Source: CAD feature listing. Evaluate the final solid. Frame: model axes, mm. A direction names the side the tool comes from. Give positions to 0.01 mm unless a question says otherwise; leave off trailing zeros. Order: outer loops, then holes, each group sorted by start corner. A loop starts at its lowest first (then second) coordinate and runs counter-clockwise, first axis right, second up.
1) Draft query along X for faces 3 (the face through (29.124, 42.853, 0.254)), 4 (the face through (75.257, 50.505, 0.254)), 5 (the face through (58, 179, 0)). Return one class per face: released by +X, released by -X, zero draft, split by the parting line, or undercut.
2) Section D-D, the plane x = 124.5. Return loops of the section in (y, z) (1 decimal).
3) Section C-C, the plane z = 5.5. Return loops of the section in (x, y) (1 decimal), plus the area to 3 significant figures.
4) Section B-B, the plane y = 129.5. Return loops of the section in (x, z), plus the area to 3 significant figures.
5) Section A-A, the plane x = 30.75. Return loops of the section in (y, z) (3 decimals).
6) Access query for faces 1 (the face through (63.4, 363.045, 0.3)), 2 (the face through (56, 179, 0.5)). Directions: +Z, -Z, +X, -X, +Y, -Y. A direction counts if a zero-diameter tool reaches every point of the face in a straight line with its end or side. Return the directions, or none.
7) First-contact query: P1, Ø1.8, axis at x = 3.175, y = 359.87, coming from the -Z side; P2, Ø1.5, axis at y = 87.5, z = 8.5, coming from the -X side; P3, Ø4, axis at x = 110.325, y = 3.35, coming from the +Z side; P4, Ø2, axis at y = 106, z = 9.5, coming from the +X side. Flat tips, straight axial feed; report the tip coordinate or a pass-through.
8) Material intervals for line 1 (Y direction, x = 30.75, z = 0.25) (3 decimals); line 2 (X direction, y = 359.87, z = 0.3) (3 decimals); line 3 (Z direction, x = 113.5, y = 111.5), sorted ascending.
Autodesk Inventor part; units mm, degrees
ref_plane "YZ Plane" through (0, 0, 0) normal (1, 0, 0) x (0, 1, 0)
ref_plane "XZ Plane" through (0, 0, 0) normal (0, 1, 0) x (-1, 0, 0)
ref_plane "XY Plane" through (0, 0, 0) normal (0, 0, 1) x (1, 0, 0)
sketch "Sketch1" plane through (0, 0, 0) normal (0, 0, 1) x (1, 0, 0)
  line L0 (0, 0) -> (113.5, 0)
  line L1 (113.5, 0) -> (113.5, 338.525)
  line L2 (113.5, 338.525) -> (0, 338.525)
  line L3 (0, 338.525) -> (0, 0)
  dimension "d0" = 113.5
  dimension "d1" = 338.525
extrude "Plate1" add sketch "Sketch1" along normal blind 0.5
sketch "Sketch2" plane through (114.0764, 338.525, 0.6152) normal (0.3842953, 0, -0.9232102) x (0, 1, 0)
  line L0 (-338.525, 0) -> (0, 0)
  line L1 (0, 0) -> (0, 29.6214)
  line L2 (0, 29.6214) -> (-338.525, 29.6214)
  line L3 (-338.525, 29.6214) -> (-338.525, 0)
edge flange "Flange1" height 30.021 angle 22.6 thickness 0.5 bend radius 1.5 thickness toward (0.3842953, 0, -0.9232102) relief tear relief width 0.5 relief depth 0.25 edges at (113.5, 169.2625, 0.5) wall of the first edge with corners at (114.0764, 0, 0.6152) (114.0764, 338.525, 0.6152) (141.4232, 338.525, 11.9985) (141.4232, 0, 11.9985)
bend "Bend1"
corner "Corner1"
sketch "Sketch3" plane through (-0.5764, 0, 0.6152) normal (-0.3842953, 0, -0.9232102) x (0, -1, 0)
  line L0 (-338.525, 0) -> (0, 0)
  line L1 (0, 0) -> (0, 29.6214)
  line L2 (0, 29.6214) -> (-338.525, 29.6214)
  line L3 (-338.525, 29.6214) -> (-338.525, 0)
edge flange "Flange2" height 30.021 angle 22.6 thickness 0.5 bend radius 1.5 thickness toward (-0.3842953, 0, -0.9232102) relief tear relief width 0.5 relief depth 0.25 edges at (0, 169.2625, 0.5) wall of the first edge with corners at (-0.5764, 338.525, 0.6152) (-0.5764, 0, 0.6152) (-27.9232, 0, 11.9985) (-27.9232, 338.525, 11.9985)
bend "Bend2"
corner "Corner2"
sketch "Sketch4" plane through (-27.9232, 0, 11.9985) normal (0.3842953, 0, 0.9232102) x (0.9232102, 0, -0.3842953)
  line L0 (0, 338.525) -> (0, 0)
  line L1 (0, 338.525) -> (0, 335.35) construction
  line L2 (0, 335.35) -> (3.175, 335.35) construction
  circle A0 centre (3.175, 335.35) radius 1.25
  line L3 (0, 0) -> (0, 3.175) construction
  line L4 (0, 3.175) -> (3.175, 3.175) construction
  line L5 (3.175, 3.175) -> (3.175, 3.35) construction
  circle A1 centre (3.175, 3.35) radius 1.25
  point P0 (30.39, 0)
  dimension "d23" = 3.175
  dimension "d24" = 3.175
  dimension "d25" = 2.5
  dimension "d26" = 3.175
  dimension "d27" = 3.175
  dimension "d62" = 0.175
  dimension "d63" = 2.5
extrude "Extrusion1" cut sketch "Sketch4" against normal blind 10
sketch "Sketch5" plane through (0, 0, 0.5) normal (0, 0, 1) x (1, 0, 0)
  line L0 (0, 0) -> (0, 338.525)
  line L1 (113.5, 0) -> (0, 0)
  line L2 (113.5, 338.525) -> (113.5, 0)
  line L3 (0, 338.525) -> (0, 335.35) construction
  line L4 (0, 335.35) -> (3.175, 335.35) construction
  line L5 (113.5, 338.525) -> (113.5, 335.35) construction
  line L6 (113.5, 335.35) -> (110.325, 335.35) construction
  line L7 (0, 0) -> (3.175, 0) construction
  line L8 (0, 0) -> (113.5, 0) construction
  line L9 (3.175, 0) -> (3.175, 3.175) construction
  line L10 (113.5, 0) -> (113.5, 3.175) construction
  line L11 (113.5, 3.175) -> (110.325, 3.175) construction
  circle A0 centre (3.175, 335.35) radius 1.25
  circle A1 centre (110.325, 335.35) radius 1.25
  line L12 (3.175, 3.175) -> (3.175, 3.35) construction
  line L13 (110.325, 3.175) -> (110.325, 3.35) construction
  circle A2 centre (110.325, 3.35) radius 1.25
  circle A3 centre (3.175, 3.35) radius 1.25
  dimension "d31" = 3.175
  dimension "d32" = 3.175
  dimension "d33" = 3.175
  dimension "d34" = 3.175
  dimension "d35" = 3.175
  dimension "d36" = 3.175
  dimension "d37" = 3.175
  dimension "d38" = 3.175
  dimension "d41" = 2.5
  dimension "d42" = 2.5
  dimension "d58" = 0.175
  dimension "d59" = 0.175
  dimension "d60" = 2.5
  dimension "d61" = 2.5
extrude "Extrusion2" cut sketch "Sketch5" against normal blind 10
sketch "Sketch6" plane through (141.4232, 0, 11.9985) normal (-0.3842953, 0, 0.9232102) x (0.9232102, 0, 0.3842953)
  line L0 (0, 338.525) -> (0, 335.35) construction
  line L1 (0, 0) -> (0, 338.525) construction
  line L2 (0, 335.35) -> (-3.175, 335.35) construction
  line L3 (0, 0) -> (0, 3.175) construction
  line L4 (0, 3.175) -> (-3.175, 3.175) construction
  circle A0 centre (-3.175, 335.35) radius 1.25
  line L5 (-3.175, 3.175) -> (-3.175, 3.35) construction
  circle A1 centre (-3.175, 3.35) radius 1.25
  point P0 (-135.1743, 0)
  dimension "d45" = 3.175
  dimension "d46" = 3.175
  dimension "d47" = 3.175
  dimension "d48" = 3.175
  dimension "d50" = 2.5
  dimension "d64" = 0.175
  dimension "d65" = 2.5
extrude "Extrusion3" cut sketch "Sketch6" against normal blind 10
sketch "Sketch7" plane through (0, 0, 0.5) normal (0, 0, 1) x (1, 0, 0)
  line L0 (-71.3896, 0) -> (266.456, 0)
  line L1 (266.456, 0) -> (266.456, 0.175)
  line L2 (266.456, 0.175) -> (-71.3896, 0.175)
  line L3 (-71.3896, 0.175) -> (-71.3896, 0)
  dimension "d53" = 0.175
extrude "Extrusion4" cut sketch "Sketch7" against normal blind 100 and the other way blind 100
sketch "Sketch9" plane through (-28.1153, 338.525, 11.5369) normal (0, 1, 0) x (0.9232102, 0, -0.3842953)
  line L0 (29.6214, -0.5) -> (29.6214, 0)
  line L1 (29.6214, 0) -> (0, 0)
  line L2 (0, -0.5) -> (0, 0)
  line L3 (0, -0.5) -> (29.6214, -0.5)
  point P0 (30.39, -0.1536)
extrude "Extrusion5" add sketch "Sketch9" along normal blind 30.87
sketch "Sketch10" plane through (0, 338.525, 0.5) normal (0, 1, 0) x (1, 0, 0)
  line L0 (-0.5764, -0.1152) -> (-0.7686, 0.3464)
  arc A0 (0, 0) -> (-0.5764, -0.1152) centre (0, -1.5) ccw
  line L1 (0, 0.5) -> (0, 0)
  arc A1 (0, 0.5) -> (-0.7686, 0.3464) centre (0, -1.5) ccw
extrude "Extrusion6" add sketch "Sketch10" along normal blind 30.87
sketch "Sketch11" plane through (0, 338.525, 0) normal (0, 1, 0) x (1, 0, 0)
  line L0 (0, -0.5) -> (113.5, -0.5)
  line L1 (113.5, 0) -> (113.5, -0.5)
  line L2 (113.5, 0) -> (0, 0)
  line L3 (0, 0) -> (0, -0.5)
extrude "Extrusion7" add sketch "Sketch11" along normal blind 30.87
sketch "Sketch12" plane through (113.5, 338.525, 0.5) normal (0, 1, 0) x (1, 0, 0)
  line L0 (0.7686, 0.3464) -> (0.5764, -0.1152)
  arc A0 (0.7686, 0.3464) -> (0, 0.5) centre (0, -1.5) ccw
  line L1 (0, 0.5) -> (0, 0)
  arc A1 (0.5764, -0.1152) -> (0, 0) centre (0, -1.5) ccw
  point P0 (-113.5, 0.5)
extrude "Extrusion8" add sketch "Sketch12" along normal blind 30.87
sketch "Sketch13" plane through (114.0764, 338.525, 0.6152) normal (0, 1, 0) x (0.9232102, 0, 0.3842953)
  line L0 (0, 0.5) -> (0, 0)
  line L1 (29.6214, 0) -> (0, 0)
  line L2 (29.6214, 0) -> (29.6214, 0.5)
  line L3 (29.6214, 0.5) -> (0, 0.5)
  point P0 (-105.553, -43.2711)
extrude "Extrusion9" add sketch "Sketch13" along normal blind 30.87
sketch "Sketch14" plane through (0, 0, 0.5) normal (0, 0, 1) x (1, 0, 0)
  circle A0 centre (3.175, 335.35) radius 1.25
  point P0 (0, 0)
extrude "Extrusion10" add sketch "Sketch14" against normal up to surface (0.5 mm away)
sketch "Sketch15" plane through (0, 0, 0.5) normal (0, 0, 1) x (1, 0, 0)
  circle A0 centre (110.325, 335.35) radius 1.25
  point P0 (0, 0)
extrude "Extrusion11" add sketch "Sketch15" against normal up to surface (0.5 mm away)
sketch "Sketch16" plane through (141.4232, 0.175, 11.9985) normal (-0.3842953, 0, 0.9232102) x (0.9232102, 0, 0.3842953)
  circle A0 centre (-3.175, 335.175) radius 1.25
  point P0 (-135.1743, -0.175)
extrude "Extrusion12" add sketch "Sketch16" against normal up to surface (0.5 mm away)
sketch "Sketch17" plane through (-0.5764, 0.175, 0.6152) normal (0.3842953, 0, 0.9232102) x (0.9232102, 0, -0.3842953)
  circle A0 centre (-26.4464, 335.175) radius 1.25
  point P0 (0.7686, -0.175)
extrude "Extrusion13" add sketch "Sketch17" against normal up to surface (0.5 mm away)
sketch "Sketch18" plane through (0, 0, 0.5) normal (0, 0, 1) x (1, 0, 0)
  line L0 (113.5, 0.175) -> (113.5, 369.395)
  line L1 (0, 0.175) -> (0, 369.395)
  line L2 (0, 369.395) -> (0, 359.87) construction
  line L3 (0, 359.87) -> (3.175, 359.87) construction
  circle A0 centre (3.175, 359.87) radius 1.5
  line L4 (113.5, 369.395) -> (113.5, 359.87) construction
  line L5 (113.5, 359.87) -> (110.325, 359.87) construction
  circle A1 centre (110.325, 359.87) radius 1.5
  point P0 (0, 0)
  dimension "d84" = 9.525
  dimension "d85" = 3.175
  dimension "d86" = 3
  dimension "d87" = 9.525
  dimension "d88" = 3.175
  dimension "d89" = 3
extrude "Extrusion14" cut sketch "Sketch18" against normal blind 30.87
sketch "Sketch19" plane through (-0.5764, 0.175, 0.6152) normal (0.3842953, 0, 0.9232102) x (0.9232102, 0, -0.3842953)
  line L0 (-29.6214, 369.22) -> (-29.6214, 0)
  line L1 (-29.6214, 369.22) -> (-29.6214, 359.695) construction
  line L2 (-29.6214, 359.695) -> (-26.4464, 359.695) construction
  circle A0 centre (-26.4464, 359.695) radius 1.5
  point P0 (0.7686, -0.175)
  dimension "d92" = 9.525
  dimension "d93" = 3.175
  dimension "d94" = 3
extrude "Extrusion15" cut sketch "Sketch19" against normal blind 30.87
sketch "Sketch20" plane through (141.4232, 0.175, 11.9985) normal (-0.3842953, 0, 0.9232102) x (0.9232102, 0, 0.3842953)
  line L0 (0, 0) -> (0, 369.22)
  line L1 (0, 369.22) -> (0, 359.695)
  line L2 (0, 359.695) -> (-3.175, 359.695)
  circle A0 centre (-3.175, 359.695) radius 1.5
  point P0 (-135.1743, -0.175)
  dimension "d97" = 9.525
  dimension "d98" = 3.175
  dimension "d99" = 3
extrude "Extrusion16" cut sketch "Sketch20" against normal blind 30.87
sketch "Sketch21" plane through (0, 0, 0.5) normal (0, 0, 1) x (1, 0, 0)
  line L0 (-35.0424, 369.395) -> (185.2939, 369.395)
  line L1 (185.2939, 369.395) -> (185.2939, 363.045)
  line L2 (185.2939, 363.045) -> (-35.0424, 363.045)
  line L3 (-35.0424, 363.045) -> (-35.0424, 369.395)
  point P0 (0, 0)
  dimension "d102" = 6.35
extrude "Extrusion17" cut sketch "Sketch21" against normal blind 30.87 and the other way blind 15.435
sketch "Sketch22" plane through (0, 0, 0.5) normal (0, 0, 1) x (1, 0, 0)
  line L0 (0, 0.175) -> (113.5, 0.175)
  line L1 (113.5, 0.175) -> (56.75, 0.175) construction
  line L2 (56.75, 0.175) -> (56.75, 50.175) construction
  line L3 (56.75, 50.175) -> (30.75, 50.175) construction
  circle A0 centre (30.75, 50.175) radius 7.5
  line L4 (56.75, 0.175) -> (56.75, 50.175) construction
  line L5 (56.75, 50.175) -> (82.75, 50.175) construction
  circle A1 centre (82.75, 50.175) radius 7.5
  point P0 (0, 0)
  dimension "d107" = 56.75
  dimension "d108" = 50
  dimension "d110" = 26
  dimension "d112" = 15
  dimension "d115" = 50
  dimension "d116" = 26
  dimension "d117" = 15
extrude "Extrusion18" cut sketch "Sketch22" against normal blind 10
equation "\"d2\" = Thickness"
equation "\"d3\" = BendReliefWidth"
equation "\"d4\" = BendReliefDepth"
equation "\"d5\" = MinimumRemnant"
equation "\"d6\" = TransitionRadius"
equation "\"d10\" = CornerReliefSize"
equation "\"d11\" = GapSize"
equation "\"d12\" = JacobiRadiusSize"
equation "\"d13\" = BendReliefWidth"
equation "\"d14\" = BendReliefDepth"
equation "\"d15\" = MinimumRemnant"
equation "\"d16\" = TransitionRadius"
equation "\"d20\" = CornerReliefSize"
equation "\"d21\" = GapSize"
equation "\"d22\" = JacobiRadiusSize"
equation "\"BendRadius\" = Thickness"
equation "\"BendReliefWidth\" = Thickness"
equation "\"BendReliefDepth\" = 0.5 * Thickness"
equation "\"CornerReliefSize\" = 4 * Thickness"
equation "\"MinimumRemnant\" = 2 * Thickness"
equation "\"TransitionRadius\" = BendRadius"
equation "\"JacobiRadiusSize\" = BendRadius"
equation "\"GapSize\" = Thickness"
properties part number "sideplate part 4"
From the geometry:
1. face 3: undercut
1. face 4: undercut
1. face 5: zero draft
2. outline: (0.2, 4.4) - (363, 4.4) - (363, 5) - (0.2, 5) - close
3. outline: (-13.6, 0.2) - (-12.3, 0.2) - (-12.3, 363) - (-13.6, 363) - close; (125.8, 0.2) - (127.1, 0.2) - (127.1, 363) - (125.8, 363) - close
3. area: 944 mm2
4. outline: (-28.12, 11.54) - (-0.77, 0.15) arc R2 ccw to (0, 0) - (113.5, 0) arc R2 ccw to (114.27, 0.15) - (141.62, 11.54) - (141.42, 12) - (114.08, 0.62) arc R1.5 cw to (113.5, 0.5) - (0, 0.5) arc R1.5 cw to (-0.58, 0.62) - (-27.92, 12) - close
4. area: 87.1 mm2
5. outline: (0.175, 0) - (42.675, 0) - (42.675, 0.5) - (0.175, 0.5) - close; (57.675, 0) - (363.045, 0) - (363.045, 0.5) - (57.675, 0.5) - close
6. face 1: +Z, -Z, +X, -X, +Y
6. face 2: +Z, +Y, -Y
7. P1: passes through
7. P2: stops at x = -22.62
7. P3: stops at z = 0.5
7. P4: stops at x = 139.12
8. line 1: y = 0.175 to 42.675, 57.675 to 363.045
8. line 2: x = -1.12 to 1.675, 4.675 to 108.825, 111.825 to 114.62
8. line 3: z = 0 to 0.5
